```python
from build123d import *

# Parameters (mm, degrees)
F0_R     = 6
F1_DEPTH = 2.5


with BuildPart() as f1:
    # F0 (on Top) → F1 (new body)
    with BuildSketch(Plane.XY):
        with BuildLine():
            Line((0, 640), (0, 0))
            Line((0, 0), (1076, 0))
            Line((1076, 0), (1076, 320))
            Line((1076, 320), (986, 320))
            ThreePointArc((986, 320), (971.857864, 325.857864), (966, 340))
            Line((966, 340), (966, 500))
            ThreePointArc((966, 500), (971.857864, 514.142136), (986, 520))
            Line((986, 520), (1158, 520))
            Line((1158, 520), (1158, 640))
            Line((1158, 640), (0, 640))
        make_face()
        with BuildLine():
            ThreePointArc((33, 554), (27, 560), (33, 566))
            Line((33, 566), (83, 566))
            ThreePointArc((83, 566), (89, 560), (83, 554))
            Line((83, 554), (33, 554))
        make_face(mode=Mode.SUBTRACT)
        with BuildLine():
            ThreePointArc((33, 609), (27, 615), (33, 621))
            Line((33, 621), (83, 621))
            ThreePointArc((83, 621), (89, 615), (83, 609))
            Line((83, 609), (33, 609))
        make_face(mode=Mode.SUBTRACT)
        with Locations((593, 560)):
            Circle(F0_R, mode=Mode.SUBTRACT)
        with Locations((593, 615)):
            Circle(F0_R, mode=Mode.SUBTRACT)
        with BuildLine():
            ThreePointArc((1075, 554), (1069, 560), (1075, 566))
            Line((1075, 566), (1125, 566))
            ThreePointArc((1125, 566), (1131, 560), (1125, 554))
            Line((1125, 554), (1075, 554))
        make_face(mode=Mode.SUBTRACT)
        with BuildLine():
            ThreePointArc((1075, 609), (1069, 615), (1075, 621))
            Line((1075, 621), (1125, 621))
            ThreePointArc((1125, 621), (1131, 615), (1125, 609))
            Line((1125, 609), (1075, 609))
        make_face(mode=Mode.SUBTRACT)
    extrude(amount=F1_DEPTH)


solid = f1.part
```
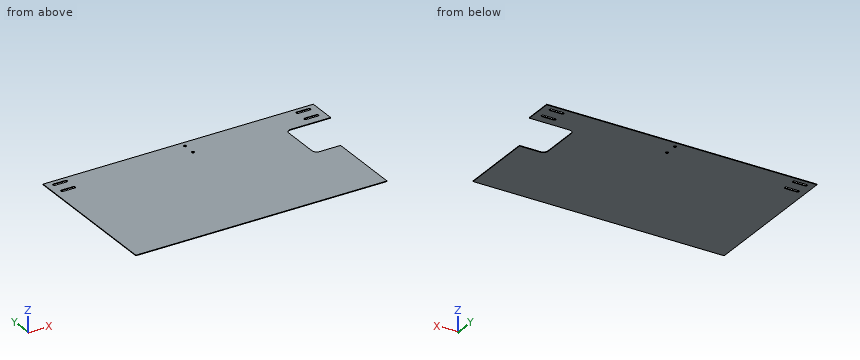
Input: part model. Units: mm. Frame: model coordinates. Give positions to 0.01 mm unless a question says otherwise; leave off trailing zeros. Order: outer loops, then holes, each group sorted by start corner. A loop starts at its lowest first (then second) coordinate and runs counter-clockwise, first axis right, second up. Notation, with made-up numbers: M 83,56 L 134,56 A24 cw 134,77 Z; hole C 6.5,25.5 d11. An arc over 180 degrees is marked long. Return JSON: item names as keys, results as strings.
1) Contact query for flat-ended pins moving along their axis: pin 1 (1.2 mm diameter, centred on x = 1088.5, z = 1, fed in from -Y); pin 2 (1.5 mm diameter, centred on y = 235.5, z = 1.5, fed in from +X). Output: stop coordinate, or through.
Taken from the geometry:
{"pin 1": "stops at y = 520", "pin 2": "stops at x = 1076"}
2) Section query B-B on z = 1.8. Output: boundary loops of the cut face in (x, y).
Taken from the geometry:
{"outline": "M 0,0 L 1076,0 L 1076,320 L 986,320 A20 cw 966,340 L 966,500 A20 cw 986,520 L 1158,520 L 1158,640 L 0,640 Z; hole M 33,554 L 83,554 A6 ccw 83,566 L 33,566 A6 ccw Z; hole M 33,609 L 83,609 A6 ccw 83,621 L 33,621 A6 ccw Z; hole C 593,560 d12; hole C 593,615 d12; hole M 1075,554 L 1125,554 A6 ccw 1125,566 L 1075,566 A6 ccw Z; hole M 1075,609 L 1125,609 A6 ccw 1125,621 L 1075,621 A6 ccw Z"}
3) Section query C-C on y = 448.5. Output: boundary loops of the cut face in (x, z).
Taken from the geometry:
{"outline": "M 0,0 L 966,0 L 966,2.5 L 0,2.5 Z"}
4) Section query A-A on x = 999. Output: boundary loops of the cut face in (y, z), and give its area (3 significant figures).
Taken from the geometry:
{"outline": "M 0,0 L 320,0 L 320,2.5 L 0,2.5 Z; M 520,0 L 640,0 L 640,2.5 L 520,2.5 Z", "area": "1,100 mm2"}
5) Line query: L1, parallel to Y at x = 593, z = 1.7; L2, parallel to X at y = 615, z = 1.8; L3, parallel to X at y = 558.5, z = 1.5. Output: solid intervals per line, ascending. Write a range as [from, to].
Taken from the geometry:
{"L1": "y = [0, 554], [566, 609], [621, 640]", "L2": "x = [0, 27], [89, 587], [599, 1069], [1131, 1158]", "L3": "x = [0, 27.19], [88.81, 587.19], [598.81, 1069.19], [1130.81, 1158]"}
6) Section query D-D on y = 77.5. Output: boundary loops of the cut face in (x, z).
Taken from the geometry:
{"outline": "M 0,0 L 1076,0 L 1076,2.5 L 0,2.5 Z"}
